Read the model definition and answer for the solid it produces. Units are mm, in the model's axes. A direction names the side the tool comes from. Give positions to 0.01 mm unless a question says otherwise; leave off trailing zeros. Write each loop counter-clockwise with the first axis right and the second up, starting at its lowest first coordinate (ties: lowest second). Pieces come first, ordered by that corner, then holes. Notation, with made-up numbers: M 65.5,42 L 73.5,42 A18 ccw 73.5,59 Z; hole C 56.5,50.5 d4. An arc over 180 degrees is marked long. Answer as CSV lines item,"result". Start each with the question number.
```python
from build123d import *

# Parameters (mm, degrees)
SKETCH1_W               = 12
SKETCH1_H               = 12
SKETCH1_R               = 4
BOSS_EXTRUDE1_DEPTH     = 4
BOSS_EXTRUDE1_2_DEPTH   = 4
BOSS_EXTRUDE1_3_DEPTH   = 4
BOSS_EXTRUDE1_4_DEPTH   = 4
BOSS_EXTRUDE1_5_DEPTH   = 4
BOSS_EXTRUDE1_6_DEPTH   = 4
BOSS_EXTRUDE2_OUTLINE_R = 1.7
BOSS_EXTRUDE2_DEPTH     = 15
SKETCH2_W               = 2.2
SKETCH2_H               = 5.00000001
SKETCH2_H_2             = 5.000000011
BOSS_EXTRUDE3_DEPTH     = 9


# Read off the part's stored shape, not the designer's step: Boss-Extrude2
with BuildPart() as part:
    # Sketch1 → Boss-Extrude1 (new body)
    with BuildSketch(Plane(origin=(0, 0, 0), x_dir=(1, 0, 0), z_dir=(0, 1, 0))):
        with Locations((3.586385956, -23.664883973)):
            Rectangle(SKETCH1_W, SKETCH1_H)
        with Locations(Location((3.586385956, -23.664883973, 0), (0, 0, 270))):
            Circle(SKETCH1_R, mode=Mode.SUBTRACT)
    extrude(amount=BOSS_EXTRUDE1_DEPTH)



with BuildPart() as body_2:
    # Sketch1 → Boss-Extrude1 2 (new body)
    with BuildSketch(Plane(origin=(0, 0, 0), x_dir=(1, 0, 0), z_dir=(0, 1, 0))):
        with Locations((-4.713614052, -10.664885052)):
            Rectangle(SKETCH1_W, SKETCH1_H)
        with Locations(Location((-4.713614052, -10.664885052, 0), (0, 0, 270))):
            Circle(SKETCH1_R, mode=Mode.SUBTRACT)
    extrude(amount=BOSS_EXTRUDE1_2_DEPTH)


with BuildPart() as body_3:
    # Sketch1 → Boss-Extrude1 3 (new body)
    with BuildSketch(Plane(origin=(0, 0, 0), x_dir=(1, 0, 0), z_dir=(0, 1, 0))):
        with Locations((11.886385948, -10.664884408)):
            Rectangle(SKETCH1_W, SKETCH1_H)
        with Locations(Location((11.886385948, -10.664884408, 0), (0, 0, 270))):
            Circle(SKETCH1_R, mode=Mode.SUBTRACT)
    extrude(amount=BOSS_EXTRUDE1_3_DEPTH)


with BuildPart() as body_4:
    # Sketch1 → Boss-Extrude1 4 (new body)
    with BuildSketch(Plane(origin=(0, 0, 0), x_dir=(1, 0, 0), z_dir=(0, 1, 0))):
        with Locations((20.186385956, -23.664884408)):
            Rectangle(SKETCH1_W, SKETCH1_H)
        with Locations(Location((20.186385956, -23.664884408, 0), (0, 0, 270))):
            Circle(SKETCH1_R, mode=Mode.SUBTRACT)
    extrude(amount=BOSS_EXTRUDE1_4_DEPTH)


with BuildPart() as body_5:
    # Sketch1 → Boss-Extrude1 5 (new body)
    with BuildSketch(Plane(origin=(0, 0, 0), x_dir=(1, 0, 0), z_dir=(0, 1, 0))):
        with Locations((28.486385948, -10.664884408)):
            Rectangle(SKETCH1_W, SKETCH1_H)
        with Locations(Location((28.486385948, -10.664884408, 0), (0, 0, 270))):
            Circle(SKETCH1_R, mode=Mode.SUBTRACT)
    extrude(amount=BOSS_EXTRUDE1_5_DEPTH)


with BuildPart() as body_6:
    # Sketch1 → Boss-Extrude1 6 (new body)
    with BuildSketch(Plane(origin=(0, 0, 0), x_dir=(1, 0, 0), z_dir=(0, 1, 0))):
        with Locations((36.786385956, -23.66488461)):
            Rectangle(SKETCH1_W, SKETCH1_H)
        with Locations(Location((36.786385956, -23.66488461, 0), (0, 0, 270))):
            Circle(SKETCH1_R, mode=Mode.SUBTRACT)
    extrude(amount=BOSS_EXTRUDE1_6_DEPTH)


with BuildPart() as part_1:
    add(part.part)

    add(body_2.part)  # Boss-Extrude2 merges body 2

    add(body_3.part)  # Boss-Extrude2 merges body 3

    add(body_4.part)  # Boss-Extrude2 merges body 4

    add(body_5.part)  # Boss-Extrude2 merges body 5

    add(body_6.part)  # Boss-Extrude2 merges body 6
    # Boss-Extrude2 outline → Boss-Extrude2 (add)
    with BuildSketch(Plane(origin=(0, 0, 0), x_dir=(1, 0, 0), z_dir=(0, 1, 0))):
        Polygon((-2.213614052, -4.164885052), (-2.213614052, -4.664885052), (1.286385948, -4.664885052), (1.286385948, -16.664885052), (-10.713614052, -16.664885052), (-10.713614052, -4.664885052), (-7.213614052, -4.664885052), (-7.213614052, -4.164885052), (-19.963614052, -4.164885052), (-19.963614052, -30.164883973), (1.086385956, -30.164883973), (1.086385956, -29.664883973), (-2.413614044, -29.664883973), (-2.413614044, -17.664883973), (9.586385956, -17.664883973), (9.586385956, -29.664883973), (6.086385956, -29.664883973), (6.086385956, -30.164883973), (17.686385956, -30.164884408), (17.686385956, -29.664884408), (14.186385956, -29.664884408), (14.186385956, -17.664884408), (26.186385956, -17.664884408), (26.186385956, -29.664884408), (22.686385956, -29.664884408), (22.686385956, -30.164884408), (34.286385956, -30.16488461), (34.286385956, -29.66488461), (30.786385956, -29.66488461), (30.786385956, -17.66488461), (42.786385956, -17.66488461), (42.786385956, -29.66488461), (39.286385956, -29.66488461), (39.286385956, -30.16488461), (52.036385956, -30.164883973), (52.036385956, -4.164885052), (30.986385948, -4.164884408), (30.986385948, -4.664884408), (34.486385948, -4.664884408), (34.486385948, -16.664884408), (22.486385948, -16.664884408), (22.486385948, -4.664884408), (25.986385948, -4.664884408), (25.986385948, -4.164884408), (14.386385948, -4.164884408), (14.386385948, -4.664884408), (17.886385948, -4.664884408), (17.886385948, -16.664884408), (5.886385948, -16.664884408), (5.886385948, -4.664884408), (9.386385948, -4.664884408), (9.386385948, -4.164884408), align=None)
        with Locations((-14.963614052, -17.164884513)):
            Circle(BOSS_EXTRUDE2_OUTLINE_R, mode=Mode.SUBTRACT)
        with Locations((47.036385956, -17.164884513)):
            Circle(BOSS_EXTRUDE2_OUTLINE_R, mode=Mode.SUBTRACT)
    extrude(amount=BOSS_EXTRUDE2_DEPTH)

    # Sketch2 → Boss-Extrude3 (add)
    with BuildSketch(Plane.XZ):
        with Locations((-0.413614044, 17.164884518)):
            Rectangle(SKETCH2_W, SKETCH2_H)
        with Locations((7.586385956, 17.164884518)):
            Rectangle(SKETCH2_W, SKETCH2_H)
        with Locations((16.186385956, 17.164884518)):
            Rectangle(SKETCH2_W, SKETCH2_H)
        with Locations((24.186385956, 17.164884518)):
            Rectangle(SKETCH2_W, SKETCH2_H)
        with Locations((32.786385956, 17.164884508)):
            Rectangle(SKETCH2_W, SKETCH2_H_2)
    extrude(amount=BOSS_EXTRUDE3_DEPTH)


solid = part_1.part
```
1. Given pin 1 (1.5 mm diameter, centred on x = 7.5, z = 21, fed in from -Y); pin 2 (3 mm diameter, centred on x = 29, y = 1.5, fed in from -Z); pin 3 (2.5 mm diameter, centred on x = 33.5, y = -4, fed in from +Z), each flat-ended and moving along its own axis, determine where each tip first touches the part or whether it passes through.
2. Determine the mould class of faces 4 (the face through (16, 9, 4.665)), 5 (the face through (-1.514, -4, 17)), 6 (the face through (33, -4, 14.665)) for opening direction X: +X half, -X half, draft (parallel to the pull), parting line (faces both ways), or undercut.
3. Find the intervals of material crossed by line 1 (X direction, y = 13.5, z = 23); line 2 (X direction, y = 4.25, z = 9.25); line 3 (Z direction, x = 41.5, y = 4.75), in increasing order. Write a range as [from, to].
4. Find section D-D on x = -15.5. Determine the outline of the cut face in (y, z), then the cut area to 3 significant figures.
5. Find section C-C on z = 21. Determine the outline of the cut face in (x, y).
6. For faces 1 (the face through (8, -4, 19.665)), 2 (the face through (23.086, -4, 17)), 3 (the face through (24, 9, 4.665)), determine the directions among +Z, -Z, +X, -X, +Y, -Y from which every point of the face is accessible in a straight line to the end or side of a thin tool.
7. Find section A-A on y = -6.25. Determine the outline of the cut face in (x, z).
8. Find section B-B on x = 47. Determine the outline of the cut face in (y, z).
Computed:
1,pin 1,"stops at y = 0"
1,pin 2,"stops at z = 4.66"
1,pin 3,"stops at z = 19.66"
2,face 4,"undercut"
2,face 5,"-X half"
2,face 6,"draft"
3,line 1,"x = [-19.96, -2.41], [9.59, 14.19], [26.19, 30.79], [42.79, 52.04]"
3,line 2,"x = [-19.96, -10.71], [1.29, 5.89], [17.89, 22.49], [34.49, 52.04]"
3,line 3,"z = [4.16, 17.66], [29.66, 30.16]"
4,outline,"M 0,4.16 L 15,4.16 L 15,15.55 L 0,15.55 Z; M 0,18.78 L 15,18.78 L 15,30.16 L 0,30.16 Z"
4,area,"342 mm^2"
5,outline,"M -19.96,0 L 0.6,0 L 0.6,4 L -2.41,4 L -2.41,15 L -19.96,15 Z; M 6.57,0 L 17.2,0 L 17.2,4 L 14.19,4 L 14.19,15 L 9.59,15 L 9.59,4 L 6.57,4 Z; M 23.17,0 L 33.8,0 L 33.8,4 L 30.79,4 L 30.79,15 L 26.19,15 L 26.19,4 L 23.17,4 Z; M 39.77,0 L 52.04,0 L 52.04,15 L 42.79,15 L 42.79,4 L 39.77,4 Z"
6,face 1,"+Z, +X, -X, -Y"
6,face 2,"+Z, -Z, -Y"
6,face 3,"+Y"
7,outline,"M -1.51,14.66 L 0.69,14.66 L 0.69,19.66 L -1.51,19.66 Z; M 6.49,14.66 L 8.69,14.66 L 8.69,19.66 L 6.49,19.66 Z; M 15.09,14.66 L 17.29,14.66 L 17.29,19.66 L 15.09,19.66 Z; M 23.09,14.66 L 25.29,14.66 L 25.29,19.66 L 23.09,19.66 Z; M 31.69,14.66 L 33.89,14.66 L 33.89,19.66 L 31.69,19.66 Z"
8,outline,"M 0,4.16 L 15,4.16 L 15,15.47 L 0,15.47 Z; M 0,18.86 L 15,18.86 L 15,30.16 L 0,30.16 Z"
